Could you check a few things on this model? Use its own coordinates, in mm. A direction names the side the tool comes from. Give positions to 0.01 mm unless a question says otherwise; leave off trailing zeros. Loops run counter-clockwise (first coordinate to the right, second up) from the corner with the lowest first, then second, coordinate; pieces in that order, holes last. Notation, with made-up numbers: (78, -30.75) - (137, -30.75) arc R12 ccw to (137, -7.75) - close; hole circle Ø2 at (71, 40.5). An arc over 180 degrees is marked (long way). Use CSV: the item, a comma, the result in double quotes.
from build123d import *

# Parameters (mm, degrees)
CROQUIS2_R              = 6
SALIENTE_EXTRUIR3_DEPTH = 10
CROQUIS9_R              = 1
SALIENTE_EXTRUIR6_DEPTH = 10


with BuildPart() as part:
    # Croquis2 → Saliente-Extruir3 (new body)
    with BuildSketch(Plane(origin=(0, 0, 0), x_dir=(1, 0, 0), z_dir=(0, 1, 0))):
        with BuildLine():
            Line((-56.772722473, 15.301893186), (-41.772722473, 15.301893186))
            ThreePointArc((-41.772722473, 15.301893186), (-34.772722473, 22.301893186), (-41.772722473, 29.301893186))
            Line((-41.772722473, 29.301893186), (-56.772722473, 29.301893186))
            Line((-56.772722473, 29.301893186), (-56.772722473, 24.301893186))
            Line((-56.772722473, 24.301893186), (-76.772722473, 24.301893186))
            Line((-76.772722473, 24.301893186), (-76.772722473, 20.301893186))
            Line((-76.772722473, 20.301893186), (-56.772722473, 20.301893186))
            Line((-56.772722473, 20.301893186), (-56.772722473, 15.301893186))
        make_face()
        with Locations((-41.772722473, 22.301893186)):
            Circle(CROQUIS2_R, mode=Mode.SUBTRACT)
    extrude(amount=SALIENTE_EXTRUIR3_DEPTH)

    # Croquis9 → Saliente-Extruir6 (add)
    with BuildSketch(Plane.XY.offset(-20.301893186)):
        with Locations((-66.52258031, 5.145347446)):
            Circle(CROQUIS9_R)
    extrude(amount=SALIENTE_EXTRUIR6_DEPTH)


solid = part.part
1) I need wall thicknesses on line 1 along Z through (x, y) = (-63, 1); line 2 along X through (y, z) = (3, -19.5); line 3 along X through (y, z) = (4, -21). Which ranges of each line are inside material? Lowest first, please.
Answer below:
line 1,"z = -24.3 to -20.3"
line 2,"x = -56.77 to -47.08, -36.47 to -35.36"
line 3,"x = -76.77 to -47.63, -35.92 to -34.89"
2) Suppose I cut it at B-B (z = -17.75). Please give me the cut outline in (x, y), plus the area to 3 significant figures.
Answer below:
outline,"circle Ø2 at (-66.52, 5.15); (-56.77, 0) - (-45.68, 0) - (-45.68, 10) - (-56.77, 10) - close; (-37.86, 0) - (-36.45, 0) - (-36.45, 10) - (-37.86, 10) - close"
area,"128 mm2"
3) I'm going to push flat-ended pins straight in: P1, Ø3, axis at x = -67.5, y = 4, coming from the -Z side; P2, Ø2, axis at x = -72, z = -17.5, coming from the -Y side; P3, Ø3, axis at x = -46.5, y = 6, coming from the +Z side. Where does each tip first touch, or does it pass through?
Answer below:
P1,"stops at z = -24.3"
P2,"passes through"
P3,"stops at z = -15.3"
4) Suppose I cut it at C-C (z = -26.5). Please give me the cut outline in (x, y), plus the area to 3 significant figures.
Answer below:
outline,"(-56.77, 0) - (-46.06, 0) - (-46.06, 10) - (-56.77, 10) - close; (-37.49, 0) - (-36.17, 0) - (-36.17, 10) - (-37.49, 10) - close"
area,"120 mm2"
5) We'd pull the mould along Z, two halves only. Please class faces 1 (the cylindrical face through (-66, 6, -15)), 2 (the cylindrical face through (-42.55, 4.93, -28.25)), 3 (the flat face through (-67, 5, -10.302)): +Z half, -Z half, draft (parallel to the pull), parting line (faces both ways), or undercut.
Answer below:
face 1,"draft"
face 2,"undercut"
face 3,"+Z half"
6) Which directions (+Z, -Z, +X, -X, +Y, -Y) give clear straight access to the entire face, cutting with the end or side of a thin tool? Please do faces 4 (the flat face through (-49, 5, -15.302)), 5 (the flat face through (-67, 5, -24.302)), 6 (the flat face through (-56.773, 5, -18)).
Answer below:
face 4,"+Z, +X, +Y, -Y"
face 5,"-Z, -X, +Y, -Y"
face 6,"+Z, +Y, -Y"
7) Suppose I cut it at D-D (y = 8.25). Please give me the cut outline in (x, z), plus the area to 3 significant figures.
Answer below:
outline,"(-76.77, -24.3) - (-56.77, -24.3) - (-56.77, -29.3) - (-41.77, -29.3) arc R7 ccw to (-41.77, -15.3) - (-56.77, -15.3) - (-56.77, -20.3) - (-76.77, -20.3) - close; hole circle Ø12 at (-41.77, -22.3)"
area,"254 mm2"
8) Suppose I cut it at A-A (x = -38). Please give me the cut outline in (y, z).
Answer below:
outline,"(0, -28.2) - (10, -28.2) - (10, -26.97) - (0, -26.97) - close; (0, -17.64) - (10, -17.64) - (10, -16.41) - (0, -16.41) - close"
